For this review, take the finished solid that the model builds, in its own axes (mm). A direction names the side the tool comes from. Give positions to 0.01 mm unless a question says otherwise; leave off trailing zeros. Write each loop counter-clockwise with the first axis right and the second up, starting at its lowest first coordinate (ties: lowest second). Pieces come first, ordered by that corner, then holes.
from build123d import *

# Parameters (mm, degrees)
BOSS_EXTRUDE_BASE_DEPTH = 6
SKETCH4_W               = 1.75
SKETCH4_H               = 40
CUT_EXTRUDE_SLOT_DEPTH  = 4.5


with BuildPart() as part:
    # Sketch1 → Boss-Extrude-Base (new body)
    with BuildSketch(Plane.XY):
        with BuildLine():
            Line((17.5, 87.375), (17.5, 10))
            ThreePointArc((17.5, 10), (14.571067812, 2.928932188), (7.5, 0))
            Line((7.5, 0), (3.5, 0))
            ThreePointArc((3.5, 0), (1.947085729, 0.204445042), (0.5, 0.803847577))
            ThreePointArc((0.5, 0.803847577), (0.133974596, 2.169872981), (1.5, 2.535898385))
            ThreePointArc((1.5, 2.535898385), (7.5, 6), (1.5, 9.464101615))
            ThreePointArc((1.5, 9.464101615), (0.133974596, 9.830127019), (0.5, 11.196152423))
            ThreePointArc((0.5, 11.196152423), (4.117292444, 11.968161362), (7.5, 10.472135955))
            Line((7.5, 10.472135955), (7.5, 46.527864045))
            ThreePointArc((7.5, 46.527864045), (4.117292444, 45.031838638), (0.5, 45.803847577))
            ThreePointArc((0.5, 45.803847577), (0.133974596, 47.169872981), (1.5, 47.535898385))
            ThreePointArc((1.5, 47.535898385), (7.5, 51), (1.5, 54.464101615))
            ThreePointArc((1.5, 54.464101615), (0.133974596, 54.830127019), (0.5, 56.196152423))
            ThreePointArc((0.5, 56.196152423), (4.117292444, 56.968161362), (7.5, 55.472135955))
            Line((7.5, 55.472135955), (7.5, 87.375))
            Line((7.5, 87.375), (17.5, 87.375))
        make_face()
    extrude(amount=BOSS_EXTRUDE_BASE_DEPTH)

    # Sketch4 → Cut-Extrude-Slot (cut)
    with BuildSketch(Plane.XY.offset(6)):
        with Locations((13.625, 64.5)):
            Rectangle(SKETCH4_W, SKETCH4_H)
    extrude(amount=-CUT_EXTRUDE_SLOT_DEPTH, mode=Mode.SUBTRACT)


solid = part.part
(1) For L1, parallel to Y at x = 3.5, z = 3.15; L2, parallel to Y at x = 13.5, z = 4 (3 decimals); L3, parallel to Y at x = 5, z = 3.45, list the stretches that pass through material, from the lowest coordinate up.
(2) We need section A-A (z = 4.1). Write out the cut boundary in (x, y) (3 decimals), and give its area (3 significant figures).
(3) The part is to be moulded in two halves that separate along Y. For faces 1 (the flat face through (7.5, 71, 3)), 2 (the cylindrical face through (0.145, 9.811, 2.958)), 3 (the cylindrical face through (1.97, 0.2, 2.96)), say which applies: +Y half, -Y half, draft (parallel to the pull), parting line (faces both ways), or undercut.
(4) We need section C-C (x = 15.25). Write out the cut boundary in (y, z) (3 decimals).
(5) We need section B-B (y = 27). Write out the cut boundary in (x, z).
(6) Tool access review of faces 4 (the flat face through (14, 84.5, 4)), 5 (the cylindrical face through (7.5, 50.9, 3)): name each direction out of +Z, -Z, +X, -X, +Y, -Y from which nothing blocks a thin tool from reaching the whole face with its end or side.
(7) Clearance check with flat-ended pins moving along their axes: pin 1 Ø2 at (y, z) = (68.5, 3) entering from -X; pin 2 Ø0.9 at (x, z) = (14, 4) entering from -Y. State where each tip first meets the part, or that it passes through.
The answers:
1. L1: y = 0 to 2, 10 to 12, 45 to 47, 55 to 57
1. L2: y = 2 to 44.5, 84.5 to 87.375
1. L3: y = 0 to 2.29, 9.71 to 11.81, 45.19 to 47.29, 54.71 to 56.81
2. outline: (0.5, 0.804) arc R6 ccw to (3.5, 0) - (7.5, 0) arc R10 ccw to (17.5, 10) - (17.5, 87.375) - (7.5, 87.375) - (7.5, 55.472) arc R6 ccw to (0.5, 56.196) arc R1 ccw to (1.5, 54.464) arc R4 cw (long way) to (1.5, 47.536) arc R1 ccw to (0.5, 45.804) arc R6 ccw to (7.5, 46.528) - (7.5, 10.472) arc R6 ccw to (0.5, 11.196) arc R1 ccw to (1.5, 9.464) arc R4 cw (long way) to (1.5, 2.536) arc R1 ccw to start; hole (12.75, 44.5) - (14.5, 44.5) - (14.5, 84.5) - (12.75, 84.5) - close
2. area: 849 mm2
3. face 1: draft
3. face 2: undercut
3. face 3: -Y half
4. outline: (3.68, 0) - (87.375, 0) - (87.375, 6) - (3.68, 6) - close
5. outline: (7.5, 0) - (17.5, 0) - (17.5, 6) - (7.5, 6) - close
6. face 4: +Z
6. face 5: +Z, -Z
7. pin 1: stops at x = 7.5
7. pin 2: stops at y = 2.04
